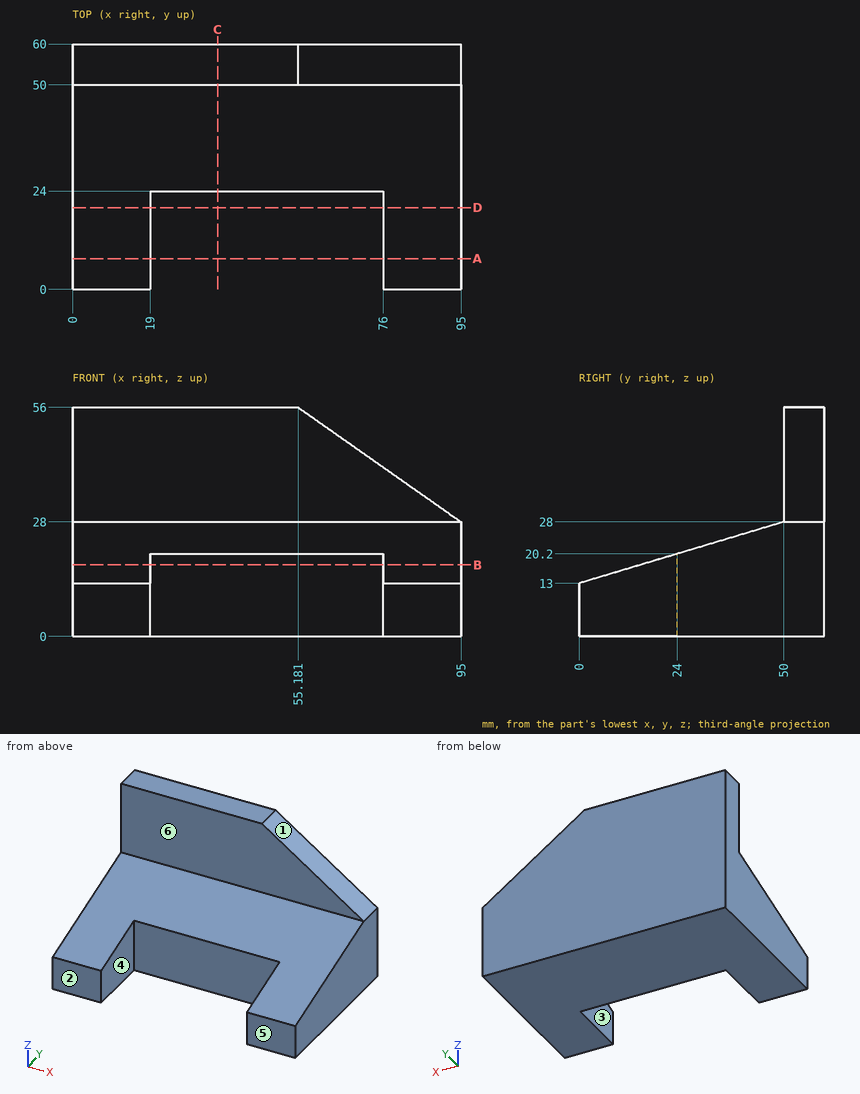
Drawing for the job (mm, zero at the part's lowest x, y, z). A direction names the side the tool comes from. Coordinates: 2 decimals unless noted, no trailing zeros. Order: outer loops, then holes, each group sorted by start corner. A loop starts at its lowest first (then second) coordinate and runs counter-clockwise, first axis right, second up. Notation, with made-up numbers: (-20, 23) - (38, 23) arc R16 cw to (38, 29) - close; hole circle Ø4 at (57.25, 23.25). An arc over 180 degrees is marked (long way). Use a Markdown table: item, result. Add a question column.
(1) Saw through at B-B (z = 17.5). Give the cut face in (x, y), then the cut area to 3 significant figures.
(2) Which spindle directions (+Z, -Z, +X, -X, +Y, -Y) get a long thin tool onto all of the face, cutting with end or side? Do the marked faces 4, 5 and 6. Say none if no direction does.
(3) Saw through at C-C (x = 35.5). Give the cut face in (y, z), then the cut area to 3 significant figures.
(4) Drill centre lines: line 1 along Y through (x, z) = (13, 52.5); line 2 along X through (y, z) = (19, 13); line 3 along Y through (x, z) = (73.5, 9). Where is each one in solid material? Low to high. Write a range as [from, to].
(5) Saw through at D-D (y = 20). Give the cut face in (x, z), then the cut area to 3 significant figures.
(6) Flat gauge pin, fed straight in: pin 1 (6 mm diameter, centred on x = 38.5, z = 7.5, fed in from -Y). Where does the tip first touch, or does it go through?
(7) Saw through at A-A (y = 7.5). Give the cut face in (x, z).
(8) Pull direction X, two halves, no side cores. Call the marked faces 1, 2 and 3: +X half, -X half, draft (parallel to the pull), parting line (faces both ways), or undercut.
Solved:
| question | item | result |
|---|---|---|
| 1 | outline | (0, 15) - (19, 15) - (19, 24) - (76, 24) - (76, 15) - (95, 15) - (95, 60) - (0, 60) - close |
| 1 | area | 3,760 mm² |
| 2 | face 4 | +Z, -Z, -Y |
| 2 | face 5 | +Z, -Z, +X, -X, -Y |
| 2 | face 6 | +Z, +X, -X, -Y |
| 3 | outline | (24, 0) - (60, 0) - (60, 56) - (50, 56) - (50, 28) - (24, 20.2) - close |
| 3 | area | 1,190 mm² |
| 4 | line 1 | y = [50, 60] |
| 4 | line 2 | x = [0, 19], [76, 95] |
| 4 | line 3 | y = [24, 60] |
| 5 | outline | (0, 0) - (19, 0) - (19, 19) - (0, 19) - close; (76, 0) - (95, 0) - (95, 19) - (76, 19) - close |
| 5 | area | 722 mm² |
| 6 | pin 1 | stops at y = 24 |
| 7 | outline | (0, 0) - (19, 0) - (19, 15.25) - (0, 15.25) - close; (76, 0) - (95, 0) - (95, 15.25) - (76, 15.25) - close |
| 8 | face 1 | +X half |
| 8 | face 2 | draft |
| 8 | face 3 | undercut |
